Here's how the part is built. I have some questions about the finished solid (model axes, mm). A direction names the side the tool comes from. Round coordinates to 2 decimals unless told otherwise and drop trailing zeros. Order: outer loops, then holes, each group sorted by start corner. A loop starts at its lowest first (then second) coordinate and runs counter-clockwise, first axis right, second up. Notation, with made-up numbers: M 81,70.5 L 120,70.5 A24 ccw 120,95.5 Z; hole C 81,-6.75 d2. An arc over 180 degrees is marked long. Write item = value, one per line. Start each with the question number.
Item 1: Please list where these lines run through material, in increasing order: L1, parallel to Y at x = -12, z = 0; L2, parallel to Z at x = 7, y = 10.5.
Item 2: I'm going to push flat-ended pins straight in: P1, Ø0.6, axis at x = 2.5, y = 10.5, coming from the +Z side; P2, Ø6, axis at y = 4.5, z = -2, coming from the +X side; P3, Ø1.5, axis at y = 9.5, z = -3.5, coming from the -X side. Where does each tip first touch, or does it pass through?
Item 3: I want a section at A-A, the plane y = 5.5. List the corners of the cut face in (x, z) for me.
Item 4: I want a section at C-C, the plane z = 4.25. List the corners of the cut face in (x, y) for me, plus the area to 3 significant figures.
Item 5: I want a section at B-B, the plane x = -7.5. List the corners of the cut face in (y, z) for me.
Item 6: For faces 1 (the face through (24.2, 10.4, 2.7)), 2 (the face through (-0.1, 10.4, -0.4)), 3 (the face through (-24.2, 10.4, -2.7)), which set-ups out of +Z, -Z, +X, -X, +Y, -Y let a thin tool reach every point of the face, with its end or its side?
```python
from build123d import *

# Parameters (mm, degrees)
SKETCH_1_R      = 0.4
EXTRUDE_1_DEPTH = 10
SKETCH_2_W      = 50
SKETCH_2_H      = 0.8
EXTRUDE_2_DEPTH = 0.8
FILLET_1_R      = 0.4
SKETCH_3_R      = 0.4
EXTRUDE_3_DEPTH = 5
SKETCH_4_R      = 0.4
EXTRUDE_4_DEPTH = 5
CHAMFER_1_SIZE  = 0.4


with BuildPart() as part:
    # 草图1 → 凸台-拉伸1 (new body)
    with BuildSketch(Plane(origin=(0, 0, 0), x_dir=(1, 0, 0), z_dir=(0, 1, 0))):
        with Locations(Location((0, 0, 0), (0, 0, 270))):
            Circle(SKETCH_1_R)
    extrude(amount=EXTRUDE_1_DEPTH)

    # 草图2 → 凸台-拉伸2 (add)
    with BuildSketch(Plane(origin=(0, 10, 0), x_dir=(1, 0, 0), z_dir=(0, 1, 0))):
        Rectangle(SKETCH_2_W, SKETCH_2_H)
    extrude(amount=EXTRUDE_2_DEPTH)

    # 圆角1
    fillet_1_edges = [part.edges().sort_by_distance(p)[0] for p in [
        (25, 10, 0),
        (25, 10.8, 0),
        (-25, 10, 0),
        (-25, 10.8, 0),
    ]]
    fillet(fillet_1_edges, radius=FILLET_1_R - 0.0001)  # a hair under: the kernel refuses the full size

    # 草图3 → 凸台-拉伸3 (add)
    with BuildSketch(Plane.XY.offset(0.4)):
        with Locations((24.6, 10.4)):
            Circle(SKETCH_3_R)
    extrude(amount=EXTRUDE_3_DEPTH)

    # 草图4 → 凸台-拉伸4 (add)
    with BuildSketch(Plane(origin=(0, 0, -0.4), x_dir=(-1, 0, 0), z_dir=(0, 0, -1))):
        with Locations((24.6, 10.4)):
            Circle(SKETCH_4_R)
    extrude(amount=EXTRUDE_4_DEPTH)

    # 倒角1
    chamfer_1_edges = [part.edges().sort_by_distance(p)[0] for p in [
        (24.2, 10.4, 5.4),
        (-24.2, 10.4, -5.4),
    ]]
    chamfer(chamfer_1_edges, length=CHAMFER_1_SIZE)


solid = part.part
```
Filled in:
q1.L1 = 10 to 10.8
q1.L2 = -0.4 to 0.4
q2.P1 = 0.4
q2.P2 = 0.4
q2.P3 = -24.97
q3.outline = C 0,0 d0.8
q4.outline = C 24.6,10.4 d0.8
q4.area = 0.503 mm^2
q5.outline = M 10,-0.4 L 10.8,-0.4 L 10.8,0.4 L 10,0.4 Z
q6.face_1 = +Z
q6.face_2 = -Z, +X, +Y, -Y
q6.face_3 = -Z
